```python
from build123d import *

# Parameters (mm, degrees)
BOSS_EXTRUDE1_DEPTH      = 19.05
BOSS_EXTRUDE1_DEPTH_BACK = 19.05
SKETCH4_W                = 186.379734437
SKETCH4_H                = 233.28599277
CUT_EXTRUDE1_DEPTH       = 950.835438404
SKETCH7_W                = 231.95079804
SKETCH7_H                = 221.677656062
CUT_EXTRUDE2_DEPTH       = 946.905059587
SKETCH11_W               = 173.814101514
SKETCH11_H               = 248.849814079
CUT_EXTRUDE4_DEPTH       = 941.51899366
SKETCH14_W               = 196.129851378
SKETCH14_H               = 225.619542635
CUT_EXTRUDE5_DEPTH       = 907.478686006
SKETCH17_W               = 176.819121146
SKETCH17_H               = 184.843776095
CUT_EXTRUDE6_DEPTH       = 913.1190158


with BuildPart() as part:
    # Sketch1 → Boss-Extrude1 (new, two sides: drawn at the far end of the back side and taken through both)
    with BuildSketch(Plane.XY.offset(-BOSS_EXTRUDE1_DEPTH_BACK)):
        with BuildLine():
            Line((832.012207401, 74.98328443), (830.051592511, 69.443138151))
            ThreePointArc((830.051592511, 69.443138151), (830.464037195, 66.534350889), (833.086070249, 65.20917293))
            Line((833.086070249, 65.20917293), (861.746459213, 65.582718771))
            ThreePointArc((861.746459213, 65.582718771), (862.436541417, 65.667855132), (863.091543165, 65.90116685))
            Line((863.091543165, 65.90116685), (872.196833975, 70.320946588))
            ThreePointArc((872.196833975, 70.320946588), (872.869650438, 70.760620145), (873.410502549, 71.355156792))
            Line((873.410502549, 71.355156792), (911.54502985, 125.773830324))
            ThreePointArc((911.54502985, 125.773830324), (913.483046359, 130.053718288), (913.732471748, 134.745320994))
            Line((913.732471748, 134.745320994), (909.364571394, 167.411013692))
            ThreePointArc((909.364571394, 167.411013692), (909.274481854, 169.840517815), (909.648990135, 172.242673089))
            Line((909.648990135, 172.242673089), (914.241820235, 190.190541175))
            ThreePointArc((914.241820235, 190.190541175), (914.334181602, 190.770696206), (914.318077922, 191.357936492))
            Line((914.318077922, 191.357936492), (911.790756949, 212.30686176))
            ThreePointArc((911.790756949, 212.30686176), (911.6522039, 212.92602807), (911.39330486, 213.505282035))
            Line((911.39330486, 213.505282035), (887.679344514, 254.884009975))
            ThreePointArc((887.679344514, 254.884009975), (882.632176652, 259.777683565), (875.755211166, 261.236892374))
            Line((875.755211166, 261.236892374), (823.370254465, 257.492913183))
            Line((823.370254465, 257.492913183), (791.391520556, 261.712016844))
            ThreePointArc((791.391520556, 261.712016844), (790.689315821, 261.726304443), (790.001151085, 261.585859009))
            Line((790.001151085, 261.585859009), (774.713390941, 256.652413374))
            ThreePointArc((774.713390941, 256.652413374), (772.534709623, 253.997511187), (774.046182712, 250.913583981))
            Line((774.046182712, 250.913583981), (788.122630404, 242.405939005))
            Line((788.122630404, 242.405939005), (863.909526126, 232.407020034))
            ThreePointArc((863.909526126, 232.407020034), (865.004538197, 232.052074317), (865.901029602, 231.330034804))
            ThreePointArc((865.901029602, 231.330034804), (881.520213, 202.699806258), (884.038410967, 170.183540241))
            ThreePointArc((884.038410967, 170.183540241), (883.978058807, 169.861693272), (883.884877802, 169.547774246))
            Line((883.884877802, 169.547774246), (869.294437604, 128.319293639))
            ThreePointArc((869.294437604, 128.319293639), (869.171364398, 128.020746389), (869.018602643, 127.736244508))
            Line((869.018602643, 127.736244508), (840.618152355, 80.745866559))
            ThreePointArc((840.618152355, 80.745866559), (840.040651792, 80.042509109), (839.287349373, 79.531868269))
            Line((839.287349373, 79.531868269), (833.618845344, 76.780331852))
            ThreePointArc((833.618845344, 76.780331852), (832.638350308, 76.040211187), (832.012207401, 74.98328443))
        make_face()
    extrude(amount=BOSS_EXTRUDE1_DEPTH + BOSS_EXTRUDE1_DEPTH_BACK)

    # Sketch4 → Cut-Extrude1 (cut, through all)
    with BuildSketch(Plane(origin=(5.154747967, 4.689434257, 78.383097783), x_dir=(0.9978522316377796, -0.003911988654162224, -0.06538822646526604), z_dir=(0.06550514342785009, 0.05959206261409093, 0.9960712134470584))):
        with Locations((842.981546385, 161.984148681)):
            Rectangle(SKETCH4_W, SKETCH4_H)
    extrude(amount=CUT_EXTRUDE1_DEPTH, mode=Mode.SUBTRACT)

    # Sketch7 → Cut-Extrude2 (cut, through all)
    with BuildSketch(Plane(origin=(9.762038751, 21.716896374, 118.29137191), x_dir=(0.9953503159229875, -0.06617162100827076, -0.06999332228967761), z_dir=(0.08090274831952654, 0.17997844984324457, 0.9803379534152342))):
        with Locations((824.773818159, 194.950225871)):
            Rectangle(SKETCH7_W, SKETCH7_H)
    extrude(amount=CUT_EXTRUDE2_DEPTH, mode=Mode.SUBTRACT)

    # Sketch11 → Cut-Extrude4 (cut, through all)
    with BuildSketch(Plane(origin=(23.549231024, 17.716627358, 158.48607319), x_dir=(0.988547763362636, -0.054240482201212636, -0.14082361180324135), z_dir=(0.14608467838170588, 0.1099028586949763, 0.983148324716462))):
        with Locations((809.66383823, 157.140332284)):
            Rectangle(SKETCH11_W, SKETCH11_H)
    extrude(amount=CUT_EXTRUDE4_DEPTH, mode=Mode.SUBTRACT)

    # Sketch14 → Cut-Extrude5 (cut, through all)
    with BuildSketch(Plane(origin=(106.606514907, -8.105609994, 291.517937711), x_dir=(0.9391673216400718, 0.019492950361294347, -0.3429063528860705), z_dir=(0.3433326783617723, -0.026104603375052715, 0.9388510114238378))):
        with Locations((805.668145938, 138.128050957)):
            Rectangle(SKETCH14_W, SKETCH14_H)
    extrude(amount=CUT_EXTRUDE5_DEPTH, mode=Mode.SUBTRACT)

    # Sketch17 → Cut-Extrude6 (cut, through all)
    with BuildSketch(Plane(origin=(107.883108977, -38.087973047, 283.754367701), x_dir=(0.9357682343427207, 0.04691042077342712, -0.34948136433573534), z_dir=(0.3526156712273392, -0.12449044441681217, 0.9274504394595959))):
        with Locations((808.154549648, 102.775727883)):
            Rectangle(SKETCH17_W, SKETCH17_H)
    extrude(amount=CUT_EXTRUDE6_DEPTH, mode=Mode.SUBTRACT)


solid = part.part
```
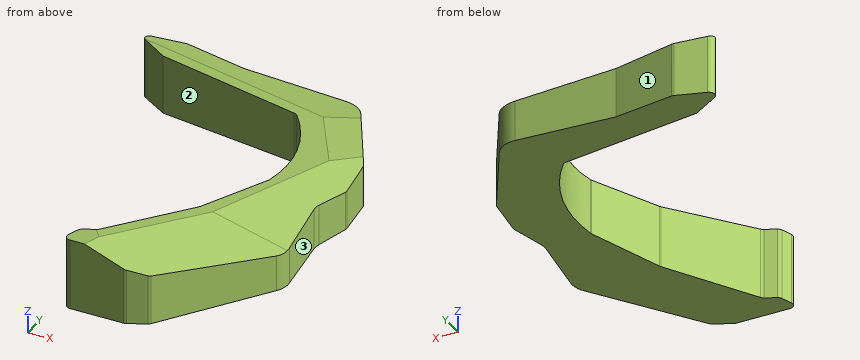
Could you check a few things on this model? Use its own coordinates, in mm. Face numbers are marked on the shaded views. A direction names the side the tool comes from. Coordinates: 2 decimals unless noted, no trailing zeros. Write each loop counter-clockwise with the first axis right and the second up, starting at its lowest first coordinate (ties: lowest second). Pieces come first, ordered by that corner, then holes. Notation, with made-up numbers: M 28.25,-1.5 L 62.25,-1.5 A25 cw 62.25,22.5 Z; hole C 70.5,27 d6. An arc over 180 degrees is marked long. Answer as CSV lines item,"result". Start each with the question number.
1) For P1, Ø5, axis at y = 201, z = -13.5, coming from the -X side; P2, Ø3, axis at x = 882.5, y = 212, coming from the +Z side; P3, Ø12, axis at x = 889.5, z = -0.5, coming from the +Y side, each with a flat end and sliding along its axis, tell me the tip position at first contact or that it passes through.
2) I want a section at A-A, the plane x = 859. Please give me the cut outline in (y, z).
3) I want a section at D-D, the plane x = 893. Please give me the cut outline in (y, z).
4) I want a section at C-C, the plane y = 184.5. Please give me the cut outline in (x, z).
5) Please list where these lines run through material, in increasing order: line 1 (Y direction, x = 840, z = -8.5); line 2 (Y direction, x = 868, z = -12); line 3 (Z direction, x = 893, y = 214). Write a range as from..to.
6) For the marked faces 1, 2 and 3, which set-ups out of +Z, -Z, +X, -X, +Y, -Y let a thin tool reach every point of the face, with its end or its side?
Data:
1,P1,"stops at x = 881.28"
1,P2,"stops at z = 8.42"
1,P3,"stops at y = 259.27"
2,outline,"M 65.55,-19.05 L 111.16,-19.05 L 111.16,15.86 L 99.04,16.59 L 65.55,12.09 Z; M 233.05,-19.05 L 260.04,-19.05 L 260.04,4.45 L 239.84,8.16 L 233.05,8.57 Z"
3,outline,"M 99.31,-19.05 L 245.6,-19.05 L 245.6,3.82 L 211.71,7.61 L 183.86,9.28 L 129.64,7.77 L 99.31,3.7 Z"
4,outline,"M 884.63,-19.05 L 912.79,-19.05 L 912.79,2.06 L 893.19,9.23 L 884.63,9.79 Z"
5,line 1,"y = 65.3..80.01, 235.56..258.68"
5,line 2,"y = 68.28..126.05, 228.78..260.68"
5,line 3,"z = -19.05..7.35"
6,face 1,"+Z, -Z, +Y"
6,face 2,"+Z, -Z, -X"
6,face 3,"+Z, -Z, +X"
